Read the model definition and answer for the solid it produces. Units are mm, in the model's axes. Round coordinates to 2 decimals unless told otherwise and drop trailing zeros. Order: outer loops, then holes, each group sorted by start corner. A loop starts at its lowest first (then second) coordinate and runs counter-clockwise, first axis right, second up. Notation, with made-up numbers: (-4.75, 31.25) -> (20.25, 31.25) arc R28 cw to (20.25, 69.25) -> close; hole circle Ø1 at (-6.5, 24.25). An arc over 180 degrees is marked (long way). Answer as a JSON object with one key per item and string values. Group by question number.
Item 1: Section B-B, the plane x = 50.5 is taken. Write down the section's boundary in (y, z).
Item 2: Consider probe 1 along X at (y, z) = (2.4, -0.5); probe 2 along X at (y, z) = (3.75, 0); probe 3 along Z at (x, y) = (64.5, 3.15). Determine where each line is inside the solid, lowest interval first. Write a range as from..to.
Item 3: Given P1, Ø1.3, axis at x = 10.88, z = 0, coming from the +Y side; P2, Ø3, axis at y = 0.5, z = 5, coming from the +X side; P3, Ø1.5, axis at x = 100.5, y = 3, coming from the +Z side, each flat-ended and moving along its own axis, determine where each tip first touches the part or whether it passes through.
Item 4: Section A-A, the plane y = 2 is taken. Write down the section's boundary in (x, z), plus the area to 3 significant figures.
Item 5: The mould has two halves that part along Z. Classify faces 1 (the cylindrical face through (142.322, 2.465, -3.855)), 2 (the cylindrical face through (-0.97, 2.46, -1.27)), 3 (the flat face through (70, 2, 4.5)), 4 (the flat face through (73, 5, 0)): pulls with the +Z half, pulls with the -Z half, needs draft (parallel to the pull), parting line crosses it, or undercut.
from build123d import *

# Parameters (mm, degrees)
SKETCH1_R           = 1.6
SKETCH1_R_2         = 0.8
BOSS_EXTRUDE1_DEPTH = 5


with BuildPart() as part:
    # Sketch1 → Boss-Extrude1 (new body)
    # profile 1 of 2: a face of its own
    with BuildSketch(Plane(origin=(0, 0, 0), x_dir=(1, 0, 0), z_dir=(0, 1, 0))):
        with BuildLine():
            Line((0, 4.5), (140, 4.5))
            ThreePointArc((140, 4.5), (144.5, 0), (140, -4.5))
            Line((140, -4.5), (0, -4.5))
            ThreePointArc((0, -4.5), (-4.5, 0), (0, 4.5))
        make_face()
        with Locations(Location((0, 0, 0), (0, 0, 270))):
            Circle(SKETCH1_R, mode=Mode.SUBTRACT)
        with Locations(Location((10.88, 0, 0), (0, 0, 270))):
            Circle(SKETCH1_R_2, mode=Mode.SUBTRACT)
        with Locations(Location((14.03, 0, 0), (0, 0, 270))):
            Circle(SKETCH1_R_2, mode=Mode.SUBTRACT)
    # profile 2 of 2: a face of its own
    with BuildSketch(Plane(origin=(0, 0, 0), x_dir=(1, 0, 0), z_dir=(0, 1, 0))):
        with BuildLine():
            Line((144.009501751, 2.043011432), (148.549527155, -6.866992459))
            ThreePointArc((148.549527155, -6.866992459), (146.583036835, -12.919505642), (140.530523653, -10.953015322))
            Line((140.530523653, -10.953015322), (135.990498249, -2.043011432))
            ThreePointArc((135.990498249, -2.043011432), (137.956988568, 4.009501751), (144.009501751, 2.043011432))
        make_face()
    extrude(amount=BOSS_EXTRUDE1_DEPTH)


solid = part.part
Values found:
{
 "1": {"outline": "(0, -4.5) -> (5, -4.5) -> (5, 4.5) -> (0, 4.5) -> close"},
 "2": {"probe 1": "-4.47..-1.52, 1.52..10.26, 11.5..13.41, 14.65..144.8", "probe 2": "-4.5..-1.6, 1.6..10.08, 11.68..13.23, 14.83..145.05", "probe 3": "-4.5..4.5"},
 "3": {"P1": "through", "P2": "x = 148.36", "P3": "z = 4.5"},
 "4": {"outline": "(0, -4.5) -> (140, -4.5) arc R4.5 ccw to (144.01, -2.04) -> (148.55, 6.87) arc R4.5 ccw to (140.53, 10.95) -> (137.24, 4.5) -> (0, 4.5) arc R4.5 ccw to start; hole circle Ø3.2 at (0, 0); hole circle Ø1.6 at (10.88, 0); hole circle Ø1.6 at (14.03, 0)", "area": "1,400 mm2"},
 "5": {"face 1": "pulls with the -Z half", "face 2": "undercut", "face 3": "pulls with the +Z half", "face 4": "needs draft"}
}
